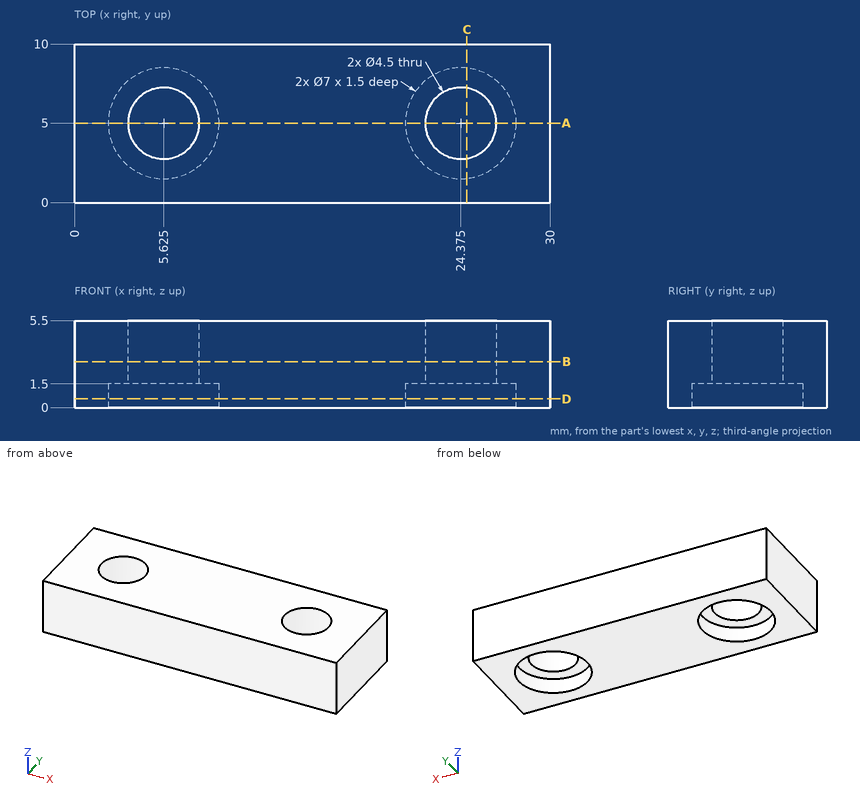
The figure shows three views and two pictorial views of one solid part (mm, origin at its lowest corner). Answer the questions. Give positions to 0.01 mm unless a question says otherwise; leave off trailing zeros. Order: outer loops, then holes, each group sorted by start corner. A loop starts at its lowest first (then second) coordinate and runs counter-clockwise, first axis right, second up. Notation, with made-up numbers: (81.5, 11) -> (99.5, 11) arc R21 cw to (99.5, 37) -> close; hole circle Ø6 at (-22.75, 39.5). An arc over 180 degrees is marked (long way). Answer as a JSON object with one key per item and string values. Group by question number.
Item 1: A flat-ended cylindrical pin translates along its axis: pin 1 (3.5 mm diameter, centred on x = 6, y = 6.5, fed in from -Z). Find the tip coordinate at first contact, or state that the pin passes through.
Item 2: The part is cut by section D-D on z = 0.55. Write down the section's boundary in (x, y) (3 decimals), and give its area (3 significant figures).
Item 3: Consider L1, parallel to X at y = 6.5, z = 1.8; L2, parallel to X at y = 6.25, z = 3.15; L3, parallel to Z at x = 23, y = 8. Determine where each line is inside the solid, lowest interval first. Write a range as from..to.
Item 4: The part is cut by section B-B on z = 2.9. Write down the section's boundary in (x, y) (3 decimals), and give its area (3 significant figures).
Item 5: The part is cut by section C-C on x = 24.75. Write down the section's boundary in (y, z), and give its area (3 significant figures).
Item 6: The part is cut by section A-A on y = 5. Write down the section's boundary in (x, z) (3 decimals), and give its area (3 significant figures).
Result set:
{
 "1": {"pin 1": "z = 1.5"},
 "2": {"outline": "(0, 0) -> (30, 0) -> (30, 10) -> (0, 10) -> close; hole circle Ø7 at (5.625, 5); hole circle Ø7 at (24.375, 5)", "area": "223 mm²"},
 "3": {"L1": "0..3.95, 7.3..22.7, 26.05..30", "L2": "0..3.75, 7.5..22.5, 26.25..30", "L3": "1.5..5.5"},
 "4": {"outline": "(0, 0) -> (30, 0) -> (30, 10) -> (0, 10) -> close; hole circle Ø4.5 at (5.625, 5); hole circle Ø4.5 at (24.375, 5)", "area": "268 mm²"},
 "5": {"outline": "(0, 0) -> (1.52, 0) -> (1.52, 1.5) -> (2.78, 1.5) -> (2.78, 5.5) -> (0, 5.5) -> close; (7.22, 1.5) -> (8.48, 1.5) -> (8.48, 0) -> (10, 0) -> (10, 5.5) -> (7.22, 5.5) -> close", "area": "26.8 mm²"},
 "6": {"outline": "(0, 0) -> (2.125, 0) -> (2.125, 1.5) -> (3.375, 1.5) -> (3.375, 5.5) -> (0, 5.5) -> close; (7.875, 1.5) -> (9.125, 1.5) -> (9.125, 0) -> (20.875, 0) -> (20.875, 1.5) -> (22.125, 1.5) -> (22.125, 5.5) -> (7.875, 5.5) -> close; (26.625, 1.5) -> (27.875, 1.5) -> (27.875, 0) -> (30, 0) -> (30, 5.5) -> (26.625, 5.5) -> close", "area": "108 mm²"}
}
